Work out the finished part from the listing and answer in its coordinate system (mm). A direction names the side the tool comes from. Round coordinates to 2 decimals unless told otherwise and drop trailing zeros. Loops run counter-clockwise (first coordinate to the right, second up) from the corner with the lowest first, then second, coordinate; pieces in that order, holes last. Notation, with made-up numbers: M 4.5,-20.75 L 36.5,-20.75 A20 ccw 36.5,-5.75 Z; hole C 61,-30 d8. An arc over 180 degrees is marked long. One line per item, written item: value.
Autodesk Inventor part; units mm, degrees
ref_plane "YZ Plane" through (0, 0, 0) normal (1, 0, 0) x (0, 1, 0)
ref_plane "XZ Plane" through (0, 0, 0) normal (0, 1, 0) x (-1, 0, 0)
ref_plane "XY Plane" through (0, 0, 0) normal (0, 0, 1) x (1, 0, 0)
sketch "草圖1" plane through (0, 0, 0) normal (0, 0, 1) x (1, 0, 0)
  circle A0 centre (0, 0) radius 4.53
  dimension "d0" = 9.06
extrude "擠出1" add sketch "草圖1" along normal blind 3.3
sketch "草圖2" plane through (0, 0, 0) normal (0, 0, -1) x (-1, 0, 0)
  line L0 (2.9402, 1.1992) -> (-2.9402, 1.1992)
  line L1 (-2.9402, -1.2408) -> (2.9402, -1.2408)
  arc A0 (-2.9402, 1.1992) -> (-2.9402, -1.2408) centre (-2.9402, -0.0208) ccw
  arc A1 (2.9402, -1.2408) -> (2.9402, 1.1992) centre (2.9402, -0.0208) ccw
  line L2 (-4.16, 0) -> (4.16, 0) construction
  arc A2 (2.9402, -0.7408) -> (2.9402, 0.6992) centre (2.9402, -0.0208) ccw
  line L3 (2.9402, 0.6992) -> (-2.9402, 0.6992)
  arc A3 (-2.9402, 0.6992) -> (-2.9402, -0.7408) centre (-2.9402, -0.0208) ccw
  line L4 (-2.9402, -0.7408) -> (2.9402, -0.7408)
  point P0 (0, 0)
  point P1 (0, 0)
  dimension "d3" = 8.32
  dimension "d5" = 2.44
  dimension "d6" = 0.5
extrude "擠出2" add sketch "草圖2" along normal blind 6.8
fillet "圓角1" radius 0.1 8 edges at (4.1602, -0.0208, -6.8) (0, -1.2408, -6.8) (-4.1602, -0.0208, -6.8) (0, 1.1992, -6.8) (-3.6602, -0.0208, -6.8) (0, -0.7408, -6.8) (3.6602, -0.0208, -6.8) (0, 0.6992, -6.8)
properties part number "磁吸頭"
1) For faces 4 (the face through (4.16, -0.05, -3.3)), 5 (the face through (3.66, -0.04, -3.3)), 6 (the face through (-4.16, 0.01, -3.3)), determine the directions among +Z, -Z, +X, -X, +Y, -Y from which every point of the face is accessible in a straight line to the end or side of a thin tool.
Check values:
face 4: -Z, +X
face 5: -Z
face 6: -Z, -X
2) Find section D-D (y = 2). Give the vertices of the cut face in (x, z), then the cut area to 3 significant figures.
Check values:
outline: M -4.06,0 L 4.06,0 L 4.06,3.3 L -4.06,3.3 Z
area: 26.8 mm2
3) Find section C-C (x = 2.5). Give the vertices of the cut face in (y, z).
Check values:
outline: M -3.78,0 L -1.24,0 L -1.24,-6.7 A0.1 ccw -1.14,-6.8 L -0.84,-6.8 A0.1 ccw -0.74,-6.7 L -0.74,0 L 0.7,0 L 0.7,-6.7 A0.1 ccw 0.8,-6.8 L 1.1,-6.8 A0.1 ccw 1.2,-6.7 L 1.2,0 L 3.78,0 L 3.78,3.3 L -3.78,3.3 Z
4) Find the intervals of material crossed by probe 1 along Y at (x, z) = (-3, -3); probe 2 along Z at (x, y) = (-1.75, -1.5); probe 3 along Y at (x, z) = (3.5, -6), in increasing order. Write a range as from..to.
Check values:
probe 1: -1.24..-0.74, 0.7..1.2
probe 2: 0..3.3
probe 3: -1.1..-0.47, 0.43..1.06
5) Find section A-A (z = -3.25). Give the vertices of the cut face in (x, y).
Check values:
outline: M -2.94,-1.24 L 2.94,-1.24 A1.22 ccw 2.94,1.2 L -2.94,1.2 A1.22 ccw Z; hole M -2.94,-0.74 L 2.94,-0.74 A0.72 ccw 2.94,0.7 L -2.94,0.7 A0.72 ccw Z
6) Find section B-B (x = 0). Give the vertices of the cut face in (y, z).
Check values:
outline: M -4.53,0 L -1.24,0 L -1.24,-6.7 A0.1 ccw -1.14,-6.8 L -0.84,-6.8 A0.1 ccw -0.74,-6.7 L -0.74,0 L 0.7,0 L 0.7,-6.7 A0.1 ccw 0.8,-6.8 L 1.1,-6.8 A0.1 ccw 1.2,-6.7 L 1.2,0 L 4.53,0 L 4.53,3.3 L -4.53,3.3 Z
7) The mould has two halves that part along X. Classify faces 1 (the face through (0, 1.199, -3)), 2 (the face through (-0.59, -4.49, 1.63)), 3 (the face through (0, 0, 0)): +X half, -X half, draft (parallel to the pull), parting line (faces both ways), or undercut.
Check values:
face 1: draft
face 2: parting line
face 3: undercut
8) Each of these flat-tipped pins is pushed along its axis until it touches: pin 1 (4 mm diameter, centred on x = -3.5, z = 0, fed in from +Y); pin 2 (3 mm diameter, centred on x = -1, z = -5, fed in from +Y); pin 3 (3 mm diameter, centred on x = -0.5, z = -2.5, fed in from -Y). Where does it stop, or does it pass through?
Check values:
pin 1: y = 4.27
pin 2: y = 1.2
pin 3: y = -1.24
